```python
from build123d import *

# Parameters (mm, degrees)
SKETCH2_R                               = 7.5
BOSS_EXTRUDE1_DEPTH                     = 10
CBORE_FOR_M5_HEX_HEAD_BOLT1_D           = 10
CBORE_FOR_M5_HEX_HEAD_BOLT1_CBORE_D     = 14
CBORE_FOR_M5_HEX_HEAD_BOLT1_CBORE_DEPTH = 10
CIRPATTERN1_COUNT                       = 4


with BuildPart() as part:
    # Sketch1 → Revolve1 (revolve)
    with BuildSketch(Plane(origin=(0, 0, 0), x_dir=(1, 0, 0), z_dir=(0, 1, 0))):
        Polygon((0, 255), (19.9, 255), (19.9, 115), (30, 115), (30, 85), (19.9, 85), (19.9, 20), (47.5, 20), (47.5, 0), (0, 0), align=None)
    revolve(axis=Axis((0, 0, 0), (0, 0, -1)))

    # Sketch2 → Boss-Extrude1 (add)
    with BuildSketch(Plane(origin=(0, 30, 0), x_dir=(1, 0, 0), z_dir=(0, 1, 0))):
        with BuildLine():
            Line((0, 115), (58.75, 115))
            ThreePointArc((58.75, 115), (70.608856816, 104.835079022), (62.376989895, 91.561252503))
            Line((62.376989895, 91.561252503), (60, 90.807558243))
            Line((60, 90.807558243), (41.684208051, 85))
            Line((41.684208051, 85), (30, 85))
            Line((30, 85), (0, 85))
            Line((0, 85), (0, 115))
        make_face()
        with Locations(Location((55, 103, 0), (0, 0, 270))):
            Circle(SKETCH2_R, mode=Mode.SUBTRACT)
    boss_extrude1 = extrude(amount=-BOSS_EXTRUDE1_DEPTH)

    # Mirror1: Boss-Extrude1 across plane
    add(boss_extrude1.mirror(Plane.ZX))

    # CBORE for M5 Hex Head Bolt1 (through all)
    with Locations(Plane(origin=(0, 0, -20), x_dir=(-1, 0, 0), z_dir=(0, 0, -1))):
        with Locations((0, 38)):
            cbore_for_m5_hex_head_bolt1 = CounterBoreHole(CBORE_FOR_M5_HEX_HEAD_BOLT1_D / 2, CBORE_FOR_M5_HEX_HEAD_BOLT1_CBORE_D / 2, CBORE_FOR_M5_HEX_HEAD_BOLT1_CBORE_DEPTH)

    # CirPattern1: CBORE for M5 Hex Head Bolt1 ×4 about axis
    cirpattern1_axis = Axis((0, 0, 0), (0, 0, 1))
    for i in range(1, CIRPATTERN1_COUNT):
        add(cbore_for_m5_hex_head_bolt1.rotate(cirpattern1_axis, i * 360 / CIRPATTERN1_COUNT), mode=Mode.SUBTRACT)


solid = part.part
```
CAD build for the part. Positions are in the model's coordinates, mm. A direction names the side the tool comes from. Round coordinates to 2 decimals unless told otherwise and drop trailing zeros. Order: outer loops, then holes, each group sorted by start corner. A loop starts at its lowest first (then second) coordinate and runs counter-clockwise, first axis right, second up.
Item 1: Pin check, flat tips, straight feed: pin 1 (11 mm diameter, centred on x = -39, y = -0.5, fed in from -Z); pin 2 (9 mm diameter, centred on x = 0, y = 38, fed in from +Z); pin 3 (4 mm diameter, centred on x = -0.5, y = 24, fed in from +Z); pin 4 (12 mm diameter, centred on y = -26, z = -99.5, fed in from -X). Stop position of each tip, or through.
Item 2: Saw through at A-A on x = -38. Write the cut outline in (y, z), then the cut area to 3 significant figures.
Item 3: Mould opens along X. For faces 1 (the face through (70.57, 25.07, -105.07)), 2 (the face through (-42.957, -0.651, -4.93)), 3 (the face through (-15.8, 12.1, -184)), 4 (the face through (-1, -1, 0)) say: pulls with the +X half, pulls with the -X half, needs draft (parallel to the pull), parting line crosses it, or undercut.
Item 4: Probe line 1 along Y through (x, z) = (0, -15); line 2 along Z through (x, y) = (17.5, -14). List the from-to ranges inside material, lowest first.
Item 5: Saw through at D-D on y = 23.5. Write the cut outline in (x, z).
Item 6: Tool access for faces 5 (the face through (-20.4, -0.7, -20)), 6 (the face through (28, 30, -100)), 7 (the face through (0.91, 44.94, -15.07)): list every direction of +Z, -Z, +X, -X, +Y, -Y with a clear straight run to the whole face (end or side of a thin tool).
Item 7: Saw through at C-C on z = -103. Write the cut outline in (x, y).
Reported:
1. pin 1: stops at z = -10
1. pin 2: passes through
1. pin 3: stops at z = 0
1. pin 4: stops at x = -22.36
2. outline: (-28.5, -20) - (-7, -20) - (-7, -10) - (-5, -10) - (-5, 0) - (-28.5, 0) - close; (5, -10) - (7, -10) - (7, -20) - (28.5, -20) - (28.5, 0) - (5, 0) - close
2. area: 900 mm2
3. face 1: pulls with the +X half
3. face 2: undercut
3. face 3: parting line crosses it
3. face 4: needs draft
4. line 1: y = -47.5 to -45, -31 to 31, 45 to 47.5
4. line 2: z = -115 to -85, -20 to 0
5. outline: (-41.28, -20) - (41.28, -20) - (41.28, 0) - (-41.28, 0) - close; (-18.65, -115) - (58.75, -115) arc R12 ccw to (62.38, -91.56) - (41.68, -85) - (-18.65, -85) - close; hole circle Ø15 at (55, -103)
6. face 5: none
6. face 6: -Z, +X, -X, +Y
6. face 7: -Z
7. outline: (0, -30) - (47.5, -30) - (47.5, -20) - (22.36, -20) arc R30 ccw to (22.36, 20) - (47.5, 20) - (47.5, 30) - (0, 30) arc R30 ccw to start; (62.5, -30) - (70.75, -30) - (70.75, -20) - (62.5, -20) - close; (62.5, 20) - (70.75, 20) - (70.75, 30) - (62.5, 30) - close
